from build123d import *

# Parameters (mm, degrees)
ESQUISSE2_R             = 1.75
BOSS_EXTRU_1_DEPTH      = 5
ESQUISSE3_R             = 39
ENL_V_MAT_EXTRU_1_DEPTH = 6


with BuildPart() as part:
    # Esquisse2 → Boss.-Extru.1 (new body)
    with BuildSketch(Plane.XY):
        with BuildLine():
            Line((0, 0), (27.5, 47.631397208))
            ThreePointArc((27.5, 47.631397208), (0, 55), (-27.5, 47.631397208))
            Line((-27.5, 47.631397208), (0, 0))
        make_face()
        with Locations((-9, 47.148700937)):
            Circle(ESQUISSE2_R, mode=Mode.SUBTRACT)
        with Locations((9, 47.148700937)):
            Circle(ESQUISSE2_R, mode=Mode.SUBTRACT)
    extrude(amount=BOSS_EXTRU_1_DEPTH)

    # Esquisse3 → Enlèv. mat.-Extru.1 (cut, through all)
    with BuildSketch(Plane(origin=(0, 0, 0), x_dir=(-1, 0, 0), z_dir=(0, 0, -1))):
        Circle(ESQUISSE3_R)
    extrude(amount=-ENL_V_MAT_EXTRU_1_DEPTH, mode=Mode.SUBTRACT)


solid = part.part
Part model, mm, in its own coordinate system. Coordinates: 2 decimals unless noted, no trailing zeros. Loops run counter-clockwise (first coordinate to the right, second up) from the corner with the lowest first, then second, coordinate; pieces in that order, holes last. Notation, with made-up numbers: (32, 86.25) -> (44, 86.25) arc R32 cw to (44, 114.25) -> close; hole circle Ø10 at (19, -20.5). An arc over 180 degrees is marked (long way). Use a Markdown table: item, result. Add a question column.
Item 1: Flat gauge pins, fed straight in: P1, Ø1.5, axis at x = 14, z = 2, coming from the +Y side; P2, Ø3, axis at x = -9, y = 47.15, coming from the -Z side; P3, Ø2, axis at x = -5, z = 1, coming from the -Y side; P4, Ø1.5, axis at x = 1.5, z = 3.5, coming from the +Y side. Where does each tip first touch, or does it go through?
Item 2: Probe probe 1 along X at (y, z) = (48.75, 4.2); probe 2 along X at (y, z) = (46.25, 0.8); probe 3 along Y at (x, z) = (-0.5, 4.5). List the from-to ranges inside material, lowest first.
Item 3: Band-saw the part on B-B on z = 1.8. Write the cut outline in (x, y) (3 decimals).
Item 4: Band-saw the part on A-A on x = 9. Write the cut outline in (y, z).
Item 5: Band-saw the part on C-C on y = 50.75. Write the cut outline in (x, z), plus the area to 3 significant figures.
Item 6: Band-saw the part on D-D on x = -8. Write the cut outline in (y, z), plus the area to 3 significant figures.
Geometry says:
| question | item | result |
|---|---|---|
| 1 | P1 | y = 53.38 |
| 1 | P2 | through |
| 1 | P3 | y = 38.54 |
| 1 | P4 | y = 54.99 |
| 2 | probe 1 | -25.46 to -9.71, -8.29 to 8.29, 9.71 to 25.46 |
| 2 | probe 2 | -26.7 to -10.5, -7.5 to 7.5, 10.5 to 26.7 |
| 2 | probe 3 | 39 to 55 |
| 3 | outline | (-27.5, 47.631) -> (-19.5, 33.775) arc R39 cw to (19.5, 33.775) -> (27.5, 47.631) arc R55 ccw to start; hole circle Ø3.5 at (-9, 47.149); hole circle Ø3.5 at (9, 47.149) |
| 4 | outline | (37.95, 0) -> (45.4, 0) -> (45.4, 5) -> (37.95, 5) -> close; (48.9, 0) -> (54.26, 0) -> (54.26, 5) -> (48.9, 5) -> close |
| 5 | outline | (-21.2, 0) -> (21.2, 0) -> (21.2, 5) -> (-21.2, 5) -> close |
| 5 | area | 212 mm² |
| 6 | outline | (38.17, 0) -> (45.71, 0) -> (45.71, 5) -> (38.17, 5) -> close; (48.58, 0) -> (54.42, 0) -> (54.42, 5) -> (48.58, 5) -> close |
| 6 | area | 66.9 mm² |
